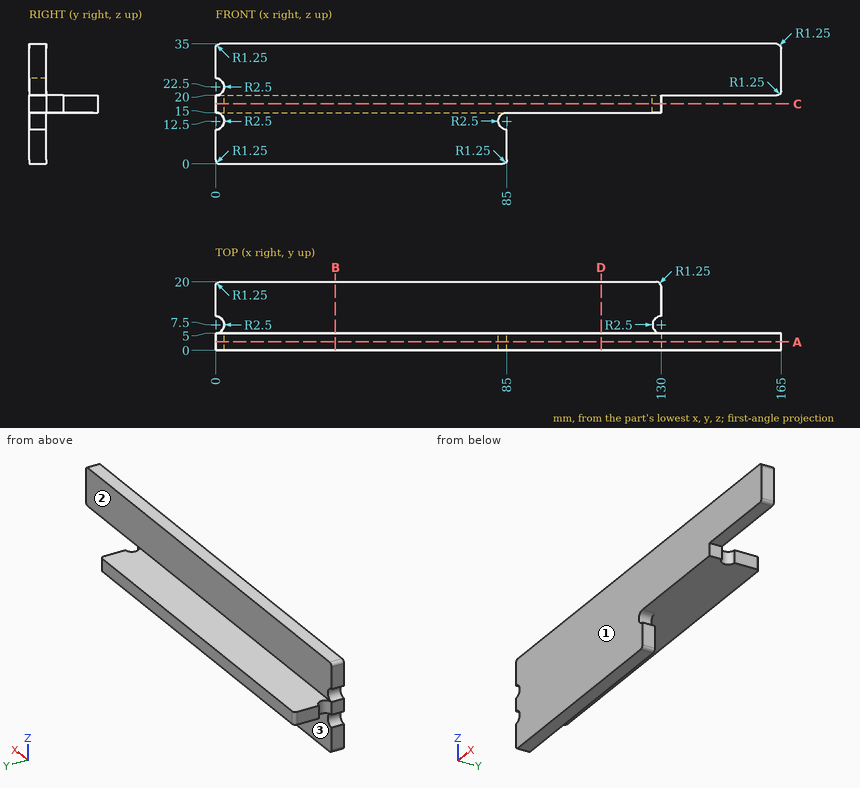
The figure shows three views and two pictorial views of one solid part (mm, origin at its lowest corner). Answer the questions. A direction names the side the tool comes from. Coordinates: 2 decimals unless noted, no trailing zeros. Order: outer loops, then holes, each group sorted by start corner. A loop starts at its lowest first (then second) coordinate and runs counter-clockwise, first axis right, second up.
Q1. Given P1, Ø4, axis at y = 2, z = 7.5, coming from the +X side; P2, Ø5.5, axis at y = 15.5, z = 18, coming from the +X side; P3, Ø4, axis at x = 115.5, z = 12, coming from the +Y side; P4, Ø12, axis at x = 96.5, y = 15, coming from the +Z side, each flat-ended and moving along its own axis, determine where each tip first touches the part or whether it passes through.
Q2. Consider line 1 (Z direction, x = 113, y = 14.5); line 2 (Y direction, x = 148.5, z = 28.5); line 3 (X direction, y = 12.25, z = 18). Determine where each line is inside the solid, lowest interval first.
Q3. A cutting plane is placed at C-C, the plane z = 17.5. Write down the section's boundary in (x, y).
Q4. A cutting plane is placed at D-D, the plane x = 112.5. Write down the section's boundary in (y, z), and give its area (3 significant figures).
Q5. A cutting plane is placed at B-B, the plane x = 35. Write down the section's boundary in (y, z).
Q6. A cutting plane is placed at A-A, the plane y = 2.5. Write down the section's boundary in (x, z), and give its area (3 significant figures).
Q7. Which of the six approach directions +Z, -Z, +X, -X, +Y, -Y give full straight-line access (tool end or side, diameter ignored) to the marked faces 1, 2 and 3?
Answers follow:
1. P1: stops at x = 85
1. P2: stops at x = 130
1. P3: passes through
1. P4: stops at z = 20
2. line 1: z = 15 to 20
2. line 2: y = 0 to 5
2. line 3: x = 0 to 130
3. outline: (0, 0) - (130, 0) - (130, 5) arc R2.5 cw to (130, 10) - (130, 18.75) arc R1.25 ccw to (128.75, 20) - (1.25, 20) arc R1.25 ccw to (0, 18.75) - (0, 10) arc R2.5 cw to (0, 5) - close
4. outline: (0, 15) - (20, 15) - (20, 20) - (5, 20) - (5, 35) - (0, 35) - close
4. area: 175 mm2
5. outline: (0, 0) - (5, 0) - (5, 15) - (20, 15) - (20, 20) - (5, 20) - (5, 35) - (0, 35) - close
6. outline: (0, 1.25) arc R1.25 ccw to (1.25, 0) - (83.75, 0) arc R1.25 ccw to (85, 1.25) - (85, 10) arc R2.5 cw to (85, 15) - (130, 15) - (130, 20) - (163.75, 20) arc R1.25 ccw to (165, 21.25) - (165, 33.75) arc R1.25 ccw to (163.75, 35) - (1.25, 35) arc R1.25 ccw to (0, 33.75) - (0, 25) arc R2.5 cw to (0, 20) - (0, 15) arc R2.5 cw to (0, 10) - close
6. area: 4,370 mm2
7. face 1: +Z, -Z, +X, -X, -Y
7. face 2: +Z, +X, -X, +Y
7. face 3: -Z, +X, -X, +Y
